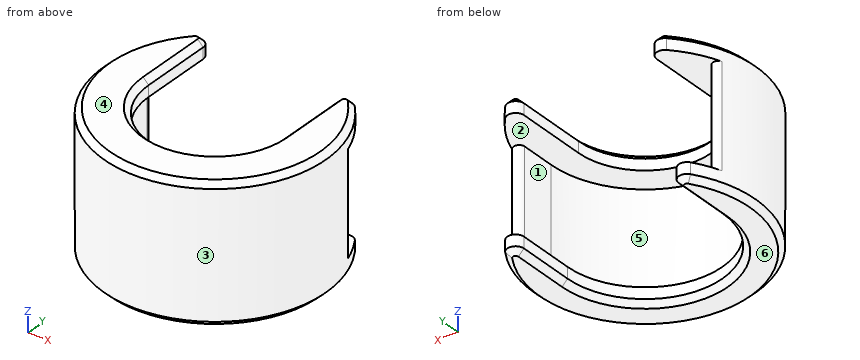
from build123d import *

# Parameters (mm, degrees)
POCKET003_DEPTH = 20.001
FILLET_R        = 1.5
FILLET001_R     = 1
CHAMFER001_SIZE = 1


with BuildPart() as part:
    # Sketch013 → Revolution003 (revolve)
    with BuildSketch(Plane.XZ):
        Polygon((-76.645, -50.35), (-76.645, -47.35), (-84.645, -47.35), (-84.645, -71.85), (-78.645, -71.85), (-78.645, -68.85), (-81.645, -68.85), (-81.645, -50.35), align=None)
    revolve(axis=Axis((-64.645, 0, -50.35), (0, 0, 1)))

    # Sketch014 → Pocket003 (cut, through all)
    with BuildSketch(Plane.XZ):
        Polygon((-76.645, -47.35), (-52.645, -47.35), (-52.645, -50.35), (-47.645, -50.35), (-47.645, -68.85), (-50.645, -68.85), (-50.645, -71.85), (-78.645, -71.85), (-78.645, -68.85), (-81.645, -68.85), (-81.645, -50.35), (-76.645, -50.35), align=None)
    extrude(amount=-POCKET003_DEPTH, mode=Mode.SUBTRACT)

    # Fillet
    fillet_edges = [part.edges().sort_by_distance(p)[0] for p in [
        (-52.645, 16, -48.85),
        (-76.645, 16, -48.85),
        (-78.645, 14.282857, -70.35),
        (-50.645, 14.282857, -70.35),
    ]]
    fillet(fillet_edges, radius=FILLET_R)

    # Fillet001
    fillet001_edges = [part.edges().sort_by_distance(p)[0] for p in [
        (-47.645, 10.535654, -59.6),
        (-81.645, 10.535654, -59.6),
    ]]
    fillet(fillet001_edges, radius=FILLET001_R)

    # Chamfer001
    chamfer001_edges = [part.edges().sort_by_distance(p)[0] for p in [
        (-83.244622, 7.352146, -47.35),
        (-83.817052, 5.694948, -71.85),
    ]]
    chamfer(chamfer001_edges, length=CHAMFER001_SIZE)


solid = part.part
Verification items for the finished model (mm, model axes). Face numbers are marked on the shaded views. A direction names the side the tool comes from. Round coordinates to 2 decimals unless told otherwise and drop trailing zeros. Loops run counter-clockwise (first coordinate to the right, second up) from the corner with the lowest first, then second, coordinate; pieces in that order, holes last. Notation, with made-up numbers: (-16.5, -39) - (-8.5, -39) arc R12 ccw to (-8.5, -32) - close; hole circle Ø4 at (56, 18). An arc over 180 degrees is marked (long way). Use a Markdown table: item, result. Add a question column.
1. Release check for a two-part mould opening along X. For the marked faces 1, 2, 3 and 4 record: released by +X, released by -X, zero draft, split by the parting line, or undercut.
2. Section check A-A, the plane z = -49. Record the boundary of the cut face in (x, y) (3 decimals).
3. Section check B-B, the plane z = -68. Record the boundary of the cut face in (x, y) (3 decimals), plus the area to 3 significant figures.
4. Gauge pin test, flat ends, axial feed: pin 1 (2 mm diameter, centred on x = -49.5, z = -62, fed in from -Y); pin 2 (2 mm diameter, centred on y = -3, z = -53, fed in from +X); pin 3 (0.6 mm diameter, centred on y = 4, z = -49.5, fed in from +X); pin 4 (6 mm diameter, centred on y = 2, z = -66, fed in from +X) (3 decimals). Record the tip position at first contact, or that the pin passes through.
5. Access from +Z, -Z, +X, -X, +Y, -Y to the whole of each face (thin tool, end or side, straight path). Record for the marked faces 5 and 6.
6. Thickness scan on probe 1 along Z at (x, y) = (-63, -15); probe 2 along Z at (x, y) = (-68, -12); probe 3 along X at (y, z) = (-1.5, -48.5). Record the ranges inside material, lowest first. Write a range as [from, to].
Checks:
| question | item | result |
|---|---|---|
| 1 | face 1 | undercut |
| 1 | face 2 | undercut |
| 1 | face 3 | split by the parting line |
| 1 | face 4 | zero draft |
| 2 | outline | (-79.24, 13.675) arc R20 ccw (long way) to (-50.05, 13.675) arc R1.5 ccw to (-52.645, 12.649) - (-52.645, 0) arc R12 cw to (-76.645, 0) - (-76.645, 12.649) arc R1.5 ccw to start |
| 3 | outline | (-83.592, 6.403) arc R20 ccw (long way) to (-45.698, 6.403) arc R1 ccw to (-47.645, 6.083) - (-47.645, 0) arc R17 cw to (-81.645, 0) - (-81.645, 6.083) arc R1 ccw to start |
| 3 | area | 210 mm^2 |
| 4 | pin 1 | stops at y = -14.14 |
| 4 | pin 2 | stops at x = -44.75 |
| 4 | pin 3 | stops at x = -44.99 |
| 4 | pin 4 | stops at x = -44.645 |
| 5 | face 5 | +Y |
| 5 | face 6 | -Z, +X, -X, +Y, -Y |
| 6 | probe 1 | z = [-71.85, -68.85], [-50.35, -47.35] |
| 6 | probe 2 | z = [-50.35, -47.89] |
| 6 | probe 3 | x = [-84.59, -76.55], [-52.74, -44.7] |
